CAD build for the part. Positions are in the model's coordinates, mm. A direction names the side the tool comes from. Coordinates: 2 decimals unless noted, no trailing zeros. Loops run counter-clockwise (first coordinate to the right, second up) from the corner with the lowest first, then second, coordinate; pieces in that order, holes last. Notation, with made-up numbers: (-29, 2.5) -> (1, 2.5) arc R19 cw to (1, 28.5) -> close; hole circle Ø11 at (-17.75, 46). An arc over 180 degrees is marked (long way). Write each question's results on one line, items separated by ' | '.
```python
from build123d import *

# Parameters (mm, degrees)
SKETCH1_R           = 4.75
BOSS_EXTRUDE1_DEPTH = 1.75


with BuildPart() as part:
    # Sketch1 → Boss-Extrude1 (new body)
    with BuildSketch(Plane.XY):
        with BuildLine():
            Line((-29.69873918, 2.664897184), (-33, 0))
            ThreePointArc((-33, 0), (-32.769980082, -3.889525088), (-32.083126945, -7.724827859))
            Line((-32.083126945, -7.724827859), (-28.249774158, -9.542905528))
            Line((-28.249774158, -9.542905528), (-27.913894972, -10.484810604))
            Line((-27.913894972, -10.484810604), (-29.731972641, -14.318163391))
            ThreePointArc((-29.731972641, -14.318163391), (-27.837130167, -17.722702504), (-25.554221367, -20.880176492))
            Line((-25.554221367, -20.880176492), (-21.311655509, -20.854978431))
            Line((-21.311655509, -20.854978431), (-20.600361522, -21.557873064))
            Line((-20.600361522, -21.557873064), (-20.575163461, -25.800438921))
            ThreePointArc((-20.575163461, -25.800438921), (-17.390795223, -28.045681335), (-13.963988845, -29.899950092))
            Line((-13.963988845, -29.899950092), (-10.152502116, -28.036467086))
            Line((-10.152502116, -28.036467086), (-9.206673827, -28.361134373))
            Line((-9.206673827, -28.361134373), (-7.343190821, -32.172621102))
            ThreePointArc((-7.343190821, -32.172621102), (-3.5, -32.813869019), (0.391982924, -32.997671878))
            Line((0.391982924, -32.997671878), (3.017478833, -29.66498959))
            Line((3.017478833, -29.66498959), (4.010508532, -29.547125193))
            Line((4.010508532, -29.547125193), (7.343190821, -32.172621102))
            ThreePointArc((7.343190821, -32.172621102), (11.084013147, -31.082867509), (14.670317668, -29.559800059))
            Line((14.670317668, -29.559800059), (15.589811092, -25.417997089))
            Line((15.589811092, -25.417997089), (16.433360491, -24.880945498))
            Line((16.433360491, -24.880945498), (20.575163461, -25.800438921))
            ThreePointArc((20.575163461, -25.800438921), (23.472701554, -23.195522882), (26.043016078, -20.26724731))
            Line((26.043016078, -20.26724731), (25.074390068, -16.136658532))
            Line((25.074390068, -16.136658532), (25.601383863, -15.286789401))
            Line((25.601383863, -15.286789401), (29.731972641, -14.318163391))
            ThreePointArc((29.731972641, -14.318163391), (31.212333545, -10.714020473), (32.257575758, -6.960517671))
            Line((32.257575758, -6.960517671), (29.592678574, -3.659256851))
            Line((29.592678574, -3.659256851), (29.69873918, -2.664897184))
            Line((29.69873918, -2.664897184), (33, 0))
            ThreePointArc((33, 0), (32.769980082, 3.889525088), (32.083126945, 7.724827859))
            Line((32.083126945, 7.724827859), (28.249774158, 9.542905528))
            Line((28.249774158, 9.542905528), (27.913894972, 10.484810604))
            Line((27.913894972, 10.484810604), (29.731972641, 14.318163391))
            ThreePointArc((29.731972641, 14.318163391), (27.837130167, 17.722702504), (25.554221367, 20.880176492))
            Line((25.554221367, 20.880176492), (21.311655509, 20.854978431))
            Line((21.311655509, 20.854978431), (20.600361522, 21.557873064))
            Line((20.600361522, 21.557873064), (20.575163461, 25.800438921))
            ThreePointArc((20.575163461, 25.800438921), (17.390795223, 28.045681335), (13.963988845, 29.899950092))
            Line((13.963988845, 29.899950092), (10.152502116, 28.036467086))
            Line((10.152502116, 28.036467086), (9.206673827, 28.361134373))
            Line((9.206673827, 28.361134373), (7.343190821, 32.172621102))
            ThreePointArc((7.343190821, 32.172621102), (3.5, 32.813869019), (-0.391982924, 32.997671878))
            Line((-0.391982924, 32.997671878), (-3.017478833, 29.66498959))
            Line((-3.017478833, 29.66498959), (-4.010508532, 29.547125193))
            Line((-4.010508532, 29.547125193), (-7.343190821, 32.172621102))
            ThreePointArc((-7.343190821, 32.172621102), (-11.084013147, 31.082867509), (-14.670317668, 29.559800059))
            Line((-14.670317668, 29.559800059), (-15.589811092, 25.417997089))
            Line((-15.589811092, 25.417997089), (-16.433360491, 24.880945498))
            Line((-16.433360491, 24.880945498), (-20.575163461, 25.800438921))
            ThreePointArc((-20.575163461, 25.800438921), (-23.472701554, 23.195522882), (-26.043016078, 20.26724731))
            Line((-26.043016078, 20.26724731), (-25.074390068, 16.136658532))
            Line((-25.074390068, 16.136658532), (-25.601383863, 15.286789401))
            Line((-25.601383863, 15.286789401), (-29.731972641, 14.318163391))
            ThreePointArc((-29.731972641, 14.318163391), (-31.212333545, 10.714020473), (-32.257575758, 6.960517671))
            Line((-32.257575758, 6.960517671), (-29.592678574, 3.659256851))
            Line((-29.592678574, 3.659256851), (-29.69873918, 2.664897184))
        make_face()
        with BuildLine():
            Line((-24.677925359, -4), (-10.246950766, -4))
            ThreePointArc((-10.246950766, -4), (-7.778174593, -7.778174593), (-4, -10.246950766))
            Line((-4, -10.246950766), (-4, -24.677925359))
            ThreePointArc((-4, -24.677925359), (-17.67766953, -17.67766953), (-24.677925359, -4))
        make_face(mode=Mode.SUBTRACT)
        with BuildLine():
            Line((4, -24.677925359), (4, -10.246950766))
            ThreePointArc((4, -10.246950766), (7.778174593, -7.778174593), (10.246950766, -4))
            Line((10.246950766, -4), (24.677925359, -4))
            ThreePointArc((24.677925359, -4), (17.67766953, -17.67766953), (4, -24.677925359))
        make_face(mode=Mode.SUBTRACT)
        with BuildLine():
            Line((24.677925359, 4), (10.246950766, 4))
            ThreePointArc((10.246950766, 4), (7.778174593, 7.778174593), (4, 10.246950766))
            Line((4, 10.246950766), (4, 24.677925359))
            ThreePointArc((4, 24.677925359), (17.67766953, 17.67766953), (24.677925359, 4))
        make_face(mode=Mode.SUBTRACT)
        with BuildLine():
            Line((-4, 24.677925359), (-4, 10.246950766))
            ThreePointArc((-4, 10.246950766), (-7.778174593, 7.778174593), (-10.246950766, 4))
            Line((-10.246950766, 4), (-24.677925359, 4))
            ThreePointArc((-24.677925359, 4), (-17.67766953, 17.67766953), (-4, 24.677925359))
        make_face(mode=Mode.SUBTRACT)
        Circle(SKETCH1_R, mode=Mode.SUBTRACT)
    extrude(amount=BOSS_EXTRUDE1_DEPTH)


solid = part.part
```
Q1. Wall check: L1, parallel to X at y = -7, z = 1.45; L2, parallel to Y at x = 16, z = 0.3; L3, parallel to Y at x = 7, z = 1. Give the ranges that are in metal, low to high. Write a range as from..to.
Results are:
L1: -32.25..-24, -8.49..8.49, 24..32.25 | L2: -25.16..-19.21, -4..4, 19.21..28.86 | L3: -31.9..-24, -8.49..8.49, 24..32.25
Q2. Cut at B-B on y = 1. Write the cut outline in (x, z).
Results are:
outline: (-31.76, 0) -> (-4.64, 0) -> (-4.64, 1.75) -> (-31.76, 1.75) -> close; (4.64, 0) -> (32.98, 0) -> (32.98, 1.75) -> (4.64, 1.75) -> close
Q3. Pull direction X, two halves, no side cores. Call faces 5 (the cylindrical face through (-17.437, -28.017, 0.863)), 6 (the cylindrical face through (31.195, -10.766, 0.863)), 7 (the flat face through (-5.65, 30.84, 0.86)), 8 (the flat face through (0, -7, 0)): +X half, -X half, draft (parallel to the pull), parting line (faces both ways), or undercut.
Results are:
face 5: -X half | face 6: +X half | face 7: undercut | face 8: draft
Q4. Cut at C-C on z = 1.25. Give the number of separate pieces and of enclosed holes in the cut face, and give its area (3 significant figures).
Results are:
separate pieces: 1 | enclosed holes: 5 | area: 2,040 mm^2
Q5. Drop flat-ended pins along their axis: pin 1 (0.9 mm diameter, centred on y = -20, z = 1, fed in from +X); pin 2 (0.5 mm diameter, centred on x = 17.5, z = 0.5, fed in from +Y); pin 3 (0.9 mm diameter, centred on x = 17.5, z = 1, fed in from -Y). Give the stop position or say it passes through.
Results are:
pin 1: x = 26.04 | pin 2: y = 28.13 | pin 3: y = -25.22
Q6. Cut at A-A on y = 19. Write the cut outline in (x, z), and give its area (3 significant figures).
Results are:
outline: (-25.75, 0) -> (-16.25, 0) -> (-16.25, 1.75) -> (-25.75, 1.75) -> close; (-4, 0) -> (4, 0) -> (4, 1.75) -> (-4, 1.75) -> close; (16.25, 0) -> (26.98, 0) -> (26.98, 1.75) -> (16.25, 1.75) -> close | area: 49.4 mm^2
Q7. Which spindle directions (+Z, -Z, +X, -X, +Y, -Y) get a long thin tool onto all of the face, cutting with end or side? Do faces 1 (the flat face through (12.08, 28.98, 0.86)), 2 (the flat face through (17, -4, 1)), 3 (the flat face through (-31.33, 1.35, 0.86)), 4 (the flat face through (25.565, -18.231, 0.863)). Say none if no direction does.
Results are:
face 1: +Z, -Z, +Y | face 2: +Z, -Z | face 3: +Z, -Z, -X | face 4: +Z, -Z, +X
Q8. Cut at D-D on x = 27. Write the cut outline in (y, z), and give its area (3 significant figures).
Results are:
outline: (-14.96, 0) -> (18.97, 0) -> (18.97, 1.75) -> (-14.96, 1.75) -> close | area: 59.4 mm^2
